from build123d import *

# Parameters (mm, degrees)
BOSS_EXTRU_1_DEPTH      = 6
ESQUISSE2_R             = 1.5
ENL_V_MAT_EXTRU_1_DEPTH = 6


with BuildPart() as part:
    # Esquisse1 → Boss.-Extru.1 (new body)
    with BuildSketch(Plane.XY):
        with BuildLine():
            Line((-31, 1.5), (-31, 7.5))
            Line((-31, 7.5), (31, 7.5))
            Line((31, 7.5), (31, 1.5))
            Line((31, 1.5), (30.809475019, 1.5))
            ThreePointArc((30.809475019, 1.5), (25, 6), (19.190524981, 1.5))
            Line((19.190524981, 1.5), (-19.190524981, 1.5))
            ThreePointArc((-19.190524981, 1.5), (-25, 6), (-30.809475019, 1.5))
            Line((-30.809475019, 1.5), (-31, 1.5))
        make_face()
    extrude(amount=BOSS_EXTRU_1_DEPTH)

    # Esquisse2 → Enlèv. mat.-Extru.1 (cut)
    with BuildSketch(Plane(origin=(0, 7.5, 0), x_dir=(1, 0, 0), z_dir=(0, 1, 0))):
        with Locations(Location((-16, -3, 0), (0, 0, 270))):
            Circle(ESQUISSE2_R)
        with Locations(Location((16, -3, 0), (0, 0, 270))):
            Circle(ESQUISSE2_R)
    extrude(amount=-ENL_V_MAT_EXTRU_1_DEPTH, mode=Mode.SUBTRACT)


solid = part.part
Verification items for the finished model (mm, model axes). Give positions to 0.01 mm unless a question says otherwise; leave off trailing zeros. Order: outer loops, then holes, each group sorted by start corner. A loop starts at its lowest first (then second) coordinate and runs counter-clockwise, first axis right, second up. Notation, with made-up numbers: M 24.25,43 L 37.25,43 A26 ccw 37.25,82 Z; hole C -26.75,-31.5 d5. An arc over 180 degrees is marked long. Use one line per item in the form item = value. Start each with the question number.
Q1. Scan lines: line 1 along X through (y, z) = (4.65, 3); line 2 along X through (y, z) = (5, 3); line 3 along X through (y, z) = (4.65, 5.3). Record each from-to range of solid material in increasing order. Write a range as [from, to].
Q2. Section check B-B (y = 2.1). Enter the section's corners in (x, z), then the cut area to 3 significant figures.
Q3. Section check C-C (x = -16). Enter the section's corners in (y, z), then the cut area to 3 significant figures.
Q4. Mould release check, pull along Z, two halves, no side actions. Record for faces 1 (the cylindrical face through (17.265, 4.542, 3.806)), 2 (the flat face through (0, 5, 6)), 3 (the flat face through (31, 5, 3)): +Z half, -Z half, draft (parallel to the pull), parting line (faces both ways), or undercut.
Q5. Section check D-D (z = 5.4). Enter the section's corners in (x, y), then the cut area to 3 significant figures.
Q6. Section check A-A (z = 3). Enter the section's corners in (x, y).
Evaluation:
q1.line_1 = [-31, -28.79], [-21.21, -17.5], [-14.5, 14.5], [17.5, 21.21], [28.79, 31]
q1.line_2 = [-31, -28.32], [-21.68, -17.5], [-14.5, 14.5], [17.5, 21.68], [28.32, 31]
q1.line_3 = [-31, -28.79], [-21.21, 21.21], [28.79, 31]
q2.outline = M -31,0 L -30.62,0 L -30.62,6 L -31,6 Z; M -19.38,0 L 19.38,0 L 19.38,6 L -19.38,6 Z; M 30.62,0 L 31,0 L 31,6 L 30.62,6 Z; hole C -16,3 d3; hole C 16,3 d3
q2.area = 223 mm2
q3.outline = M 1.5,0 L 7.5,0 L 7.5,1.5 L 1.5,1.5 Z; M 1.5,4.5 L 7.5,4.5 L 7.5,6 L 1.5,6 Z
q3.area = 18.0 mm2
q4.face_1 = undercut
q4.face_2 = +Z half
q4.face_3 = draft
q5.outline = M -31,1.5 L -30.81,1.5 A6 cw -19.19,1.5 L 19.19,1.5 A6 cw 30.81,1.5 L 31,1.5 L 31,7.5 L -31,7.5 Z
q5.area = 295 mm2
q6.outline = M -31,1.5 L -30.81,1.5 A6 cw -19.19,1.5 L -17.5,1.5 L -17.5,7.5 L -31,7.5 Z; M -14.5,1.5 L 14.5,1.5 L 14.5,7.5 L -14.5,7.5 Z; M 17.5,1.5 L 19.19,1.5 A6 cw 30.81,1.5 L 31,1.5 L 31,7.5 L 17.5,7.5 Z
